The model under review builds one solid part; all positions refer to its coordinate system, in mm. Coordinates: 2 decimals unless noted, no trailing zeros. Answer as CSV lines item,"result". Start each with the question number.
from build123d import *

# Parameters (mm, degrees)
SKETCH2_R           = 2.05
BOSS_EXTRUDE1_DEPTH = 360
SKETCH3_R           = 2.75
CUT_EXTRUDE1_DEPTH  = 34


with BuildPart() as part:
    # Sketch2 → Boss-Extrude1 (new body)
    with BuildSketch(Plane.XY):
        with BuildLine():
            Line((-3.642230561, 1.287773026), (-3.642230561, -1.287773026))
            ThreePointArc((-3.642230561, -1.287773026), (-3.87999308, -2.483085929), (-4.55708345, -3.496423279))
            Line((-4.55708345, -3.496423279), (-7.182004606, -6.121344434))
            ThreePointArc((-7.182004606, -6.121344434), (-7.704200045, -6.225215565), (-8, -5.782519648))
            Line((-8, -5.782519648), (-8, -3.622007668))
            ThreePointArc((-8, -3.622007668), (-8.161974206, -3.230967343), (-8.553014531, -3.068993137))
            Line((-8.553014531, -3.068993137), (-9.443284204, -3.068993137))
            ThreePointArc((-9.443284204, -3.068993137), (-9.836715763, -3.229656566), (-10, -3.622007668))
            Line((-10, -3.622007668), (-10, -8.939033256))
            ThreePointArc((-10, -8.939033256), (-9.689250035, -9.689250035), (-8.939033256, -10))
            Line((-8.939033256, -10), (-3.622007668, -10))
            ThreePointArc((-3.622007668, -10), (-3.229656566, -9.836715763), (-3.068993137, -9.443284204))
            Line((-3.068993137, -9.443284204), (-3.068993137, -8.553014531))
            ThreePointArc((-3.068993137, -8.553014531), (-3.230967343, -8.161974206), (-3.622007668, -8))
            Line((-3.622007668, -8), (-5.782519648, -8))
            ThreePointArc((-5.782519648, -8), (-6.225215565, -7.704200045), (-6.121344434, -7.182004606))
            Line((-6.121344434, -7.182004606), (-3.496423279, -4.55708345))
            ThreePointArc((-3.496423279, -4.55708345), (-2.483085929, -3.87999308), (-1.287773026, -3.642230561))
            Line((-1.287773026, -3.642230561), (1.287773026, -3.642230561))
            ThreePointArc((1.287773026, -3.642230561), (2.483085929, -3.87999308), (3.496423279, -4.55708345))
            Line((3.496423279, -4.55708345), (6.121344434, -7.182004606))
            ThreePointArc((6.121344434, -7.182004606), (6.225215565, -7.704200045), (5.782519648, -8))
            Line((5.782519648, -8), (3.622007668, -8))
            ThreePointArc((3.622007668, -8), (3.230967343, -8.161974206), (3.068993137, -8.553014531))
            Line((3.068993137, -8.553014531), (3.068993137, -9.443284204))
            ThreePointArc((3.068993137, -9.443284204), (3.229656566, -9.836715763), (3.622007668, -10))
            Line((3.622007668, -10), (8.939033256, -10))
            ThreePointArc((8.939033256, -10), (9.689250035, -9.689250035), (10, -8.939033256))
            Line((10, -8.939033256), (10, -3.622007668))
            ThreePointArc((10, -3.622007668), (9.836715763, -3.229656566), (9.443284204, -3.068993137))
            Line((9.443284204, -3.068993137), (8.553014531, -3.068993137))
            ThreePointArc((8.553014531, -3.068993137), (8.161974206, -3.230967343), (8, -3.622007668))
            Line((8, -3.622007668), (8, -5.782519648))
            ThreePointArc((8, -5.782519648), (7.704200045, -6.225215565), (7.182004606, -6.121344434))
            Line((7.182004606, -6.121344434), (4.55708345, -3.496423279))
            ThreePointArc((4.55708345, -3.496423279), (3.87999308, -2.483085929), (3.642230561, -1.287773026))
            Line((3.642230561, -1.287773026), (3.642230561, 1.287773026))
            ThreePointArc((3.642230561, 1.287773026), (3.87999308, 2.483085929), (4.55708345, 3.496423279))
            Line((4.55708345, 3.496423279), (7.182004606, 6.121344434))
            ThreePointArc((7.182004606, 6.121344434), (7.704200045, 6.225215565), (8, 5.782519648))
            Line((8, 5.782519648), (8, 3.622007668))
            ThreePointArc((8, 3.622007668), (8.161974206, 3.230967343), (8.553014531, 3.068993137))
            Line((8.553014531, 3.068993137), (9.443284204, 3.068993137))
            ThreePointArc((9.443284204, 3.068993137), (9.836715763, 3.229656566), (10, 3.622007668))
            Line((10, 3.622007668), (10, 8.939033256))
            ThreePointArc((10, 8.939033256), (9.689250035, 9.689250035), (8.939033256, 10))
            Line((8.939033256, 10), (3.622007668, 10))
            ThreePointArc((3.622007668, 10), (3.229656566, 9.836715763), (3.068993137, 9.443284204))
            Line((3.068993137, 9.443284204), (3.068993137, 8.553014531))
            ThreePointArc((3.068993137, 8.553014531), (3.230967343, 8.161974206), (3.622007668, 8))
            Line((3.622007668, 8), (5.782519648, 8))
            ThreePointArc((5.782519648, 8), (6.225215565, 7.704200045), (6.121344434, 7.182004606))
            Line((6.121344434, 7.182004606), (3.496423279, 4.55708345))
            ThreePointArc((3.496423279, 4.55708345), (2.483085929, 3.87999308), (1.287773026, 3.642230561))
            Line((1.287773026, 3.642230561), (-1.287773026, 3.642230561))
            ThreePointArc((-1.287773026, 3.642230561), (-2.483085929, 3.87999308), (-3.496423279, 4.55708345))
            Line((-3.496423279, 4.55708345), (-6.121344434, 7.182004606))
            ThreePointArc((-6.121344434, 7.182004606), (-6.225215565, 7.704200045), (-5.782519648, 8))
            Line((-5.782519648, 8), (-3.622007668, 8))
            ThreePointArc((-3.622007668, 8), (-3.230967343, 8.161974206), (-3.068993137, 8.553014531))
            Line((-3.068993137, 8.553014531), (-3.068993137, 9.443284204))
            ThreePointArc((-3.068993137, 9.443284204), (-3.229656566, 9.836715763), (-3.622007668, 10))
            Line((-3.622007668, 10), (-8.939033256, 10))
            ThreePointArc((-8.939033256, 10), (-9.689250035, 9.689250035), (-10, 8.939033256))
            Line((-10, 8.939033256), (-10, 3.622007668))
            ThreePointArc((-10, 3.622007668), (-9.836715763, 3.229656566), (-9.443284204, 3.068993137))
            Line((-9.443284204, 3.068993137), (-8.553014531, 3.068993137))
            ThreePointArc((-8.553014531, 3.068993137), (-8.161974206, 3.230967343), (-8, 3.622007668))
            Line((-8, 3.622007668), (-8, 5.782519648))
            ThreePointArc((-8, 5.782519648), (-7.704200045, 6.225215565), (-7.182004606, 6.121344434))
            Line((-7.182004606, 6.121344434), (-4.55708345, 3.496423279))
            ThreePointArc((-4.55708345, 3.496423279), (-3.87999308, 2.483085929), (-3.642230561, 1.287773026))
        make_face()
        Circle(SKETCH2_R, mode=Mode.SUBTRACT)
    extrude(amount=-BOSS_EXTRUDE1_DEPTH)

    # Sketch3 → Cut-Extrude1 (cut)
    with BuildSketch(Plane(origin=(0, 10, 0), x_dir=(1, 0, 0), z_dir=(0, 1, 0))):
        with Locations(Location((0, 110, 0), (0, 0, 297.922776764))):
            Circle(SKETCH3_R)
    extrude(amount=-CUT_EXTRUDE1_DEPTH, mode=Mode.SUBTRACT)


solid = part.part
1) Mouldability with a two-part tool opening along X and no side actions: class faces 1 (the flat face through (-0.1, 2.4, 0)), 2 (the cylindrical face through (2.242, 0.056, -111.593)) as +X half, -X half, draft (parallel to the pull), parting line (faces both ways), or undercut.
2) Clearance check with a flat-ended pin moving along its axis: pin 1 Ø0.8 at (x, z) = (-0.5, -56.5) entering from -Y. State where the tip first meets the part, or that it passes through.
3) To check wall thickness, follow line 1 (X direction, y = 0, z = -166); line 2 (X direction, y = 5.25, z = -112); line 3 (X direction, y = 1.25, z = -110). State the ranges of each line that lie inside material, in increasing order. Write a range as [from, to].
Results:
1,face 1,"draft"
1,face 2,"undercut"
2,pin 1,"stops at y = -3.64"
3,line 1,"x = [-3.64, -2.05], [2.05, 3.64]"
3,line 2,"x = [-10, -8], [-6.31, -4.19], [4.19, 6.31], [8, 10]"
3,line 3,"x = [-3.64, -2.75], [2.75, 3.64]"
